Verification items for the finished model (mm, model axes). A direction names the side the tool comes from. Coordinates: 2 decimals unless noted, no trailing zeros. Order: outer loops, then holes, each group sorted by start corner. A loop starts at its lowest first (then second) coordinate and runs counter-clockwise, first axis right, second up. Notation, with made-up numbers: (-17.5, -27.75) -> (28.5, -27.75) arc R16 cw to (28.5, 0.25) -> close; hole circle Ø1 at (47.5, 13). An arc over 180 degrees is marked (long way). Use CSV: the item, a comma, the result in double quotes. Start each with the question number.
1) Release check for a two-part mould opening along Y. For faces 1 (the flat face through (0, -1, 28)), 2 (the flat face through (12, -47.5, 11)), 3 (the cylindrical face through (39.699, 37.357, 3.204)), 4 (the flat face through (12, 47.5, 11)) record: released by +Y, released by -Y, zero draft, split by the parting line, or undercut.
2) Go/stop test with flat-tipped pins: pin 1 (1.5 mm diameter, centred on y = 9.5, z = 13.5, fed in from +X); pin 2 (3 mm diameter, centred on x = 12, y = 26, fed in from +Z); pin 3 (11 mm diameter, centred on y = 36, z = 27, fed in from +X); pin 4 (17 mm diameter, centred on x = 44, y = 15, fed in from +Z). Record where each tip stops, or that it passes through.
3) Sectioned sample at D-D on y = 18. Record the boundary of the cut face in (x, z).
4) Sectioned sample at B-B on y = 39. Record the boundary of the cut face in (x, z).
5) Sectioned sample at C-C on z = 30. Record the boundary of the cut face in (x, y).
6) Scan lines: line 1 along Y through (x, z) = (4.25, 27); line 2 along X through (y, z) = (31.5, 4.5); line 3 along Y through (x, z) = (41, 2.5). Record each from-to range of solid material in increasing order.
7) Sectioned sample at A-A on x = 41. Record the boundary of the cut face in (y, z).
8) Tool access check on faces 5 (the flat face through (44, -1, 6.5)), 6 (the flat face through (61, -1, 3)). Record the directions out of +Z, -Z, +X, -X, +Y, -Y that give a thin tool (end or side, any length) a straight path to the whole face; none if there is none.
from build123d import *

# Parameters (mm, degrees)
F1_DEPTH = 47.5
F2_R     = 6
F3_DEPTH = 55.001
F4_R     = 6
F5_DEPTH = 61.001


with BuildPart() as f1:
    # F0 (on Front) → F1 (new body, symmetric)
    with BuildSketch(Plane.XZ):
        with BuildLine():
            Line((0, 55), (0, 0))
            Line((0, 0), (61, 0))
            Line((61, 0), (61, 6.5))
            Line((61, 6.5), (26.5, 6.5))
            ThreePointArc((26.5, 6.5), (12.357864, 12.357864), (6.5, 26.5))
            Line((6.5, 26.5), (6.5, 55))
            Line((6.5, 55), (0, 55))
        make_face()
    extrude(amount=F1_DEPTH, both=True)

    # F2 (on face) → F3 (cut, through all)
    with BuildSketch(Plane(origin=(0, 0, 0), x_dir=(1, 0, 0), z_dir=(0, 0, -1))):
        with Locations((41, 31.5)):
            Circle(F2_R)
        with Locations((41, -31.5)):
            Circle(F2_R)
    extrude(amount=-F3_DEPTH, mode=Mode.SUBTRACT)

    # F4 (on face) → F5 (cut, through all)
    with BuildSketch(Plane(origin=(0, 0, 0), x_dir=(0, -1, 0), z_dir=(-1, 0, 0))):
        with Locations((-36, 27)):
            Circle(F4_R)
        with Locations((36, 27.5)):
            Circle(F4_R)
        with BuildLine():
            Line((21.029741, 55), (-21.029741, 55))
            ThreePointArc((-21.029741, 55), (0, 40.5), (21.029741, 55))
        make_face()
    extrude(amount=-F5_DEPTH, mode=Mode.SUBTRACT)


solid = f1.part
Answers follow:
1,face 1,"zero draft"
1,face 2,"released by -Y"
1,face 3,"undercut"
1,face 4,"released by +Y"
2,pin 1,"stops at x = 11.98"
2,pin 2,"stops at z = 14.5"
2,pin 3,"passes through"
2,pin 4,"stops at z = 6.5"
3,outline,"(0, 0) -> (61, 0) -> (61, 6.5) -> (26.5, 6.5) arc R20 cw to (6.5, 26.5) -> (6.5, 49.5) -> (0, 49.5) -> close"
4,outline,"(0, 0) -> (61, 0) -> (61, 6.5) -> (26.5, 6.5) arc R20 cw to (7.06, 21.8) -> (0, 21.8) -> close; (0, 32.2) -> (6.5, 32.2) -> (6.5, 55) -> (0, 55) -> close"
5,outline,"(0, -47.5) -> (6.5, -47.5) -> (6.5, -41.45) -> (0, -41.45) -> close; (0, -30.55) -> (6.5, -30.55) -> (6.5, 30.8) -> (0, 30.8) -> close; (0, 41.2) -> (6.5, 41.2) -> (6.5, 47.5) -> (0, 47.5) -> close"
6,line 1,"y = -47.5 to -41.98, -30.02 to 30, 42 to 47.5"
6,line 2,"x = 0 to 35, 47 to 61"
6,line 3,"y = -47.5 to -37.5, -25.5 to 25.5, 37.5 to 47.5"
7,outline,"(-47.5, 0) -> (-37.5, 0) -> (-37.5, 6.5) -> (-47.5, 6.5) -> close; (-25.5, 0) -> (25.5, 0) -> (25.5, 6.5) -> (-25.5, 6.5) -> close; (37.5, 0) -> (47.5, 0) -> (47.5, 6.5) -> (37.5, 6.5) -> close"
8,face 5,"+Z, +X, +Y, -Y"
8,face 6,"+Z, -Z, +X, +Y, -Y"
